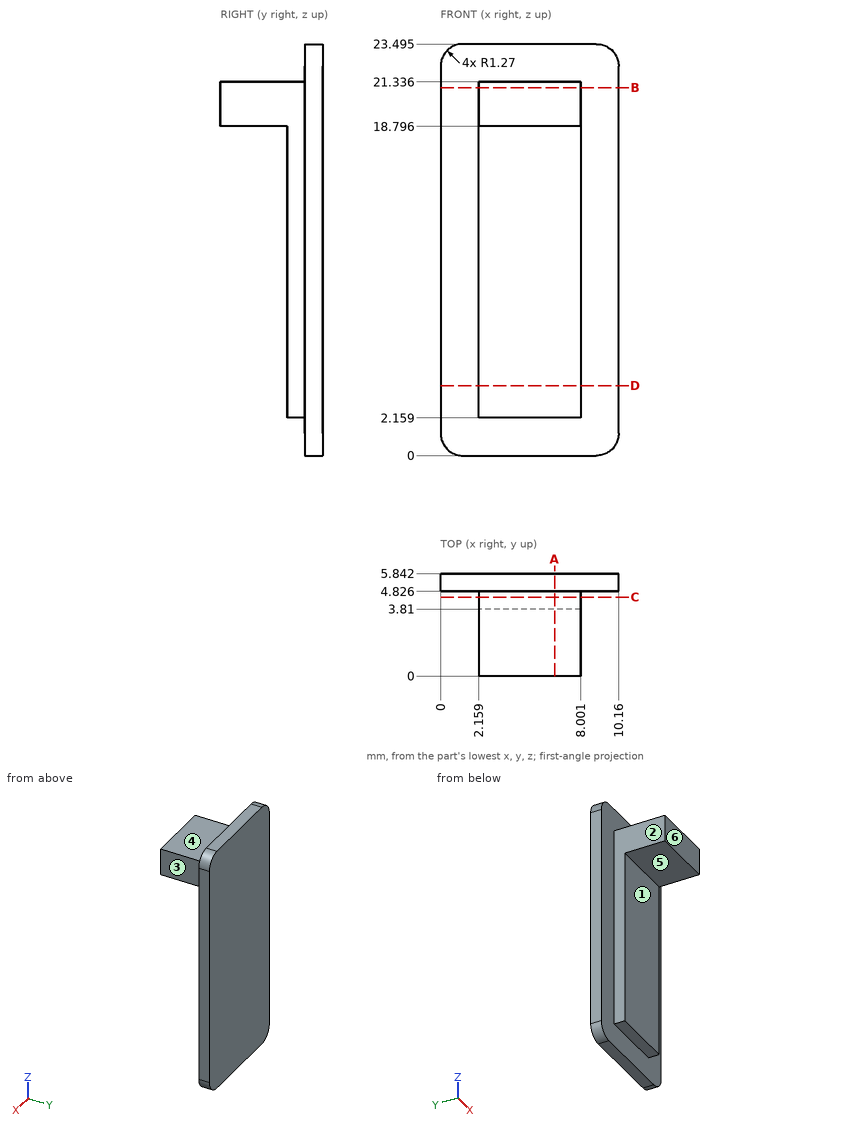
Study the drawing (mm; zero at the part's minimum x, y, z) and answer. A direction names the side the tool comes from. Give positions to 0.01 mm unless a question says otherwise; leave off trailing zeros. Write each loop counter-clockwise with the first axis right and the second up, starting at its lowest first coordinate (ties: lowest second). Pieces come first, ordered by that corner, then holes. Notation, with made-up numbers: (12.5, 27.5) -> (49.5, 27.5) arc R27 ccw to (49.5, 55.5) -> close; hole circle Ø8 at (10.5, -16). An arc over 180 degrees is marked (long way). Answer in a Markdown table with one row per item.
1) A tool of negligible diameter and unlimited length cuts with its end or side. For the marked faces 1, 2 and 3, from which of +Z, -Z, +X, -X, +Y, -Y can it reach the whole face along a straight path? Write none if from no direction.
Results list:
| item | result |
|---|---|
| face 1 | -Z, +X, -X, -Y |
| face 2 | +Z, -Z, -X, -Y |
| face 3 | +Z, -Z, +X, -Y |
2) Determine the mould class of the marked faces 4, 5 and 6 for opening direction Z: released by +Z, released by -Z, zero draft, split by the parting line, or undercut.
Results list:
| item | result |
|---|---|
| face 4 | released by +Z |
| face 5 | released by -Z |
| face 6 | zero draft |
3) Section A-A on x = 6.5 is taken. Give the vertices of the cut face in (y, z) (3 decimals), plus the area to 3 significant figures.
Results list:
| item | result |
|---|---|
| outline | (0, 18.796) -> (3.81, 18.796) -> (3.81, 2.159) -> (4.826, 2.159) -> (4.826, 0) -> (5.842, 0) -> (5.842, 23.495) -> (4.826, 23.495) -> (4.826, 21.336) -> (0, 21.336) -> close |
| area | 53.0 mm^2 |
4) Section B-B on z = 21 is taken. Give the vertices of the cut face in (x, y).
Results list:
| item | result |
|---|---|
| outline | (0, 4.83) -> (2.16, 4.83) -> (2.16, 0) -> (8, 0) -> (8, 4.83) -> (10.16, 4.83) -> (10.16, 5.84) -> (0, 5.84) -> close |
5) Straight lines are drawn through the part: line 1 (Y direction, x = 8.5, z = 10.5); line 2 (Y direction, x = 3, z = 8.5); line 3 (X direction, y = 4.25, z = 12.75). For each, find the intervals that lie inside material, in ascending order. Write a range as [from, to].
Results list:
| item | result |
|---|---|
| line 1 | [4.83, 5.84] |
| line 2 | [3.81, 5.84] |
| line 3 | [2.16, 8] |
6) Section D-D on z = 4 is taken. Give the vertices of the cut face in (x, y).
Results list:
| item | result |
|---|---|
| outline | (0, 4.83) -> (2.16, 4.83) -> (2.16, 3.81) -> (8, 3.81) -> (8, 4.83) -> (10.16, 4.83) -> (10.16, 5.84) -> (0, 5.84) -> close |
7) Each of these flat-tipped pins is pushed along its axis until it touches: pin 1 Ø5 at (x, z) = (6, 7.5) entering from -Y; pin 2 Ø1.5 at (y, z) = (4, 21) entering from +X; pin 3 Ø3 at (x, y) = (4.5, 1.5) entering from -Z. Where does it stop, or does it pass through?
Results list:
| item | result |
|---|---|
| pin 1 | y = 3.81 |
| pin 2 | x = 8 |
| pin 3 | z = 18.8 |
8) Section C-C on y = 4.5 is taken. Give the vertices of the cut face in (x, z), plus the area to 3 significant figures.
Results list:
| item | result |
|---|---|
| outline | (2.16, 2.16) -> (8, 2.16) -> (8, 21.34) -> (2.16, 21.34) -> close |
| area | 112 mm^2 |
